```python
from build123d import *

# Parameters (mm, degrees)
SKETCH1_W    = 15
SKETCH1_H    = 10
BASE_DEPTH   = 8
SPACER_DEPTH = 1.5
SKETCH4_W    = 15
SKETCH4_H    = 10
TOP_DEPTH    = 5
SKETCH5_R    = 1.6
BORE_DEPTH   = 18.073371079
NUT_DEPTH    = 2.2


with BuildPart() as part:
    # Sketch1 → base (new body)
    with BuildSketch(Plane(origin=(0, 0, 0), x_dir=(1, 0, 0), z_dir=(0, 1, 0))):
        Rectangle(SKETCH1_W, SKETCH1_H)
    extrude(amount=BASE_DEPTH)

    # Sketch3 → spacer (add)
    with BuildSketch(Plane(origin=(0, 8, 0), x_dir=(1, 0, 0), z_dir=(0, 1, 0))):
        Polygon((-7.5, 3), (-5.99621099, 3), (5.99621099, 3), (7.5, 3), (7.5, 5), (-7.5, 5), align=None)
    extrude(amount=SPACER_DEPTH)

    # Sketch4 → top (add)
    with BuildSketch(Plane(origin=(0, 9.5, 0), x_dir=(1, 0, 0), z_dir=(0, 1, 0))):
        Rectangle(SKETCH4_W, SKETCH4_H)
    extrude(amount=TOP_DEPTH)

    # Sketch5 → bore (cut, through all)
    with BuildSketch(Plane(origin=(0, 14.5, 0), x_dir=(1, 0, 0), z_dir=(0, 1, 0))):
        with Locations(Location((0, -1, 0), (0, 0, 270))):
            Circle(SKETCH5_R)
    extrude(amount=-BORE_DEPTH, mode=Mode.SUBTRACT)

    # Sketch6 → nut (cut)
    with BuildSketch(Plane(origin=(0, 14.5, 0), x_dir=(1, 0, 0), z_dir=(0, 1, 0))):
        Polygon((0, -4.1), (2.684678752, -2.55), (2.684678752, 0.55), (0, 2.1), (-2.684678752, 0.55), (-2.684678752, -2.55), align=None)
    extrude(amount=-NUT_DEPTH, mode=Mode.SUBTRACT)


solid = part.part
```
For this review, take the finished solid that the model builds, in its own axes (mm). A direction names the side the tool comes from. Round coordinates to 2 decimals unless told otherwise and drop trailing zeros. Write each loop counter-clockwise with the first axis right and the second up, starting at its lowest first coordinate (ties: lowest second). Pieces come first, ordered by that corner, then holes.
1) Take a section at D-D on z = 1. Give the boundary of the cut face in (x, y), then the cut area to 3 significant figures.
Answer below:
outline: (-7.5, 0) - (-1.6, 0) - (-1.6, 8) - (-7.5, 8) - close; (-7.5, 9.5) - (-1.6, 9.5) - (-1.6, 12.3) - (-2.68, 12.3) - (-2.68, 14.5) - (-7.5, 14.5) - close; (1.6, 0) - (7.5, 0) - (7.5, 8) - (1.6, 8) - close; (1.6, 9.5) - (7.5, 9.5) - (7.5, 14.5) - (2.68, 14.5) - (2.68, 12.3) - (1.6, 12.3) - close
area: 149 mm2
2) Take a section at C-C on x = 1. Give the boundary of the cut face in (y, z).
Answer below:
outline: (0, -5) - (14.5, -5) - (14.5, -1.52) - (12.3, -1.52) - (12.3, -0.25) - (9.5, -0.25) - (9.5, -3) - (8, -3) - (8, -0.25) - (0, -0.25) - close; (0, 2.25) - (8, 2.25) - (8, 5) - (0, 5) - close; (9.5, 2.25) - (12.3, 2.25) - (12.3, 3.52) - (14.5, 3.52) - (14.5, 5) - (9.5, 5) - close
3) Insertion check: pin 1 Ø4 at (x, z) = (0, 1) entering from +Y. The pin has a flat end and moves straight along its axis. Give the tip position at first contact, or say it passes through.
Answer below:
pin 1: stops at y = 12.3
4) For line 1 along X through (y, z) = (13.75, 0.5); line 2 along Y through (x, z) = (6.75, 1.25); line 3 along X through (y, z) = (2.75, 1), list the stretches that pass through material, from the lowest coordinate up.
Answer below:
line 1: x = -7.5 to -2.68, 2.68 to 7.5
line 2: y = 0 to 8, 9.5 to 14.5
line 3: x = -7.5 to -1.6, 1.6 to 7.5
5) Mouldability with a two-part tool opening along X and no side actions: class faces 4 (the face through (0, 12, 5)), 5 (the face through (2.685, 13, 1)), 6 (the face through (7.5, 7, 0)) as +X half, -X half, draft (parallel to the pull), parting line (faces both ways), or undercut.
Answer below:
face 4: draft
face 5: undercut
face 6: +X half
6) Take a section at A-A on z = -2.5. Give the boundary of the cut face in (x, y), then the cut area to 3 significant figures.
Answer below:
outline: (-7.5, 0) - (7.5, 0) - (7.5, 8) - (-7.5, 8) - close; (-7.5, 9.5) - (7.5, 9.5) - (7.5, 14.5) - (-7.5, 14.5) - close
area: 195 mm2
7) Machinability: for faces 1 (the face through (-2, 9.5, 1)), 2 (the face through (1.361, 13.415, -1.314)), 3 (the face through (-0.97, 10.92, -0.27)), which of the approach directions +Z, -Z, +X, -X, +Y, -Y give a long, thin tool a straight path to every point of the face, cutting with its end or side? Answer none if there is none.
Answer below:
face 1: +Z, +X, -X
face 2: +Y
face 3: +Y, -Y
8) Take a section at B-B on y = 11.75. Give the boundary of the cut face in (x, z), then the cut area to 3 significant figures.
Answer below:
outline: (-7.5, -5) - (7.5, -5) - (7.5, 5) - (-7.5, 5) - close; hole circle Ø3.2 at (0, 1)
area: 142 mm2
